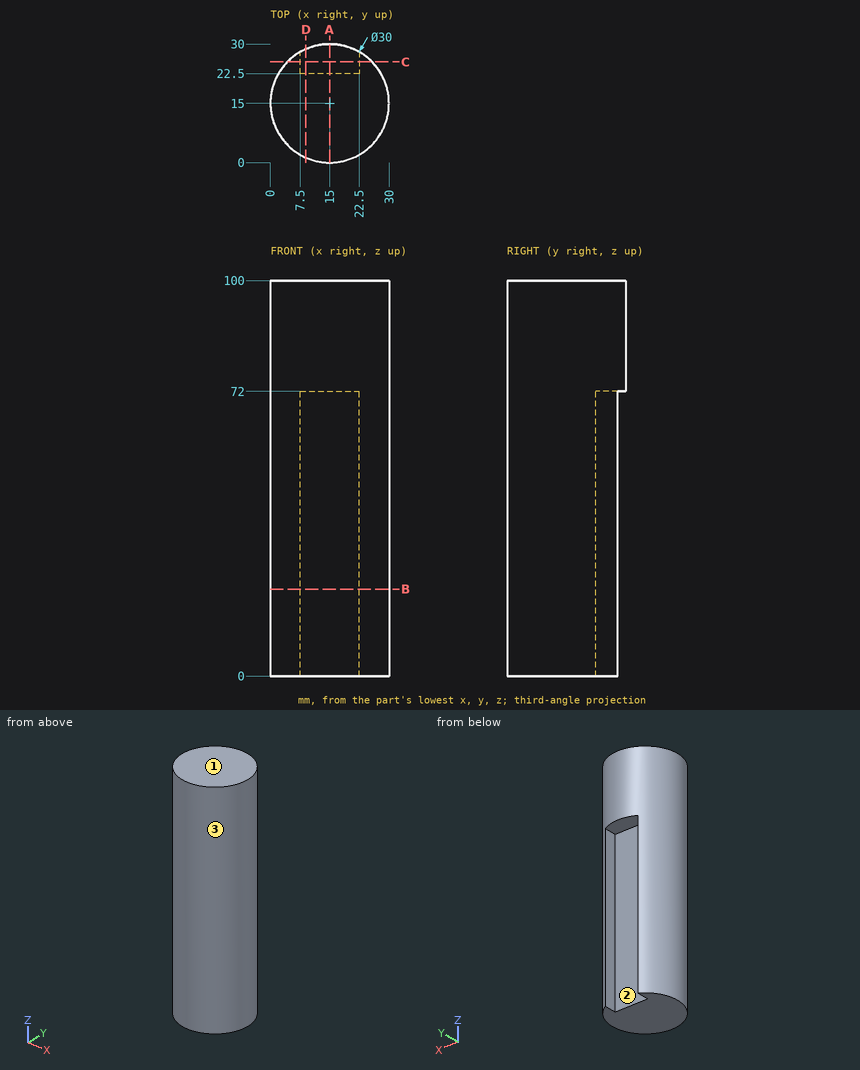
Geometry check sheet. Reference: drawing and pictorial views, mm from the part's lowest x, y, z. Give positions to 0.01 mm unless a question says otherwise; leave off trailing zeros. Write each loop counter-clockwise with the first axis right and the second up, starting at its lowest first coordinate (ties: lowest second). Pieces come first, ordered by that corner, then holes. Notation, with made-up numbers: (30.5, 82) -> (41.5, 82) arc R30 ccw to (41.5, 118) -> close; hole circle Ø6 at (88, 89.25). An arc over 180 degrees is marked (long way). One line per item, written item: value. Start each with the question number.
Item 1: Section check D-D on x = 9. Record the cut outline in (y, z).
Item 2: Section check C-C on y = 25.5. Record the cut outline in (x, z).
Item 3: Section check A-A on x = 15. Record the cut outline in (y, z), then the cut area to 3 significant figures.
Item 4: Material ranges on probe 1 along X at (y, z) = (2, 58); probe 2 along Z at (x, y) = (20.75, 23.5); probe 3 along X at (y, z) = (26, 31), recorded low to high. Write a range as from..to.
Item 5: Gauge pin test, flat ends, axial feed: pin 1 (3 mm diameter, centred on y = 4, z = 44, fed in from -X); pin 2 (1.5 mm diameter, centred on y = 13.5, z = 27.5, fed in from -X); pin 3 (3 mm diameter, centred on y = 9.5, z = 69, fed in from -X); pin 4 (10 mm diameter, centred on y = 18.5, z = 67.5, fed in from +X). Record the tip position at first contact, or that the pin passes through.
Item 6: Section check B-B on z = 22. Record the cut outline in (x, y), then the cut area to 3 significant figures.
Item 7: Draft check along X on the marked faces 1, 2 and 3. Enter one of: +X half, -X half, draft (parallel to the pull), parting line (faces both ways), or undercut.
Results list:
1. outline: (1.25, 0) -> (22.5, 0) -> (22.5, 72) -> (28.75, 72) -> (28.75, 100) -> (1.25, 100) -> close
2. outline: (4.29, 0) -> (7.5, 0) -> (7.5, 72) -> (22.5, 72) -> (22.5, 0) -> (25.71, 0) -> (25.71, 100) -> (4.29, 100) -> close
3. outline: (0, 0) -> (22.5, 0) -> (22.5, 72) -> (30, 72) -> (30, 100) -> (0, 100) -> close
3. area: 2,460 mm²
4. probe 1: 7.52..22.48
4. probe 2: 72..100
4. probe 3: 4.8..7.5, 22.5..25.2
5. pin 1: x = 3.39
5. pin 2: x = 0.02
5. pin 3: x = 0.54
5. pin 4: x = 30
6. outline: (7.5, 22.5) -> (7.5, 27.99) arc R15 ccw (long way) to (22.5, 27.99) -> (22.5, 22.5) -> close
6. area: 604 mm²
7. face 1: draft
7. face 2: undercut
7. face 3: parting line
